from build123d import *

# Parameters (mm, degrees)
SKETCH2_R               = 10
BOSS_EXTRUDE1_DEPTH     = 70
CUT_EXTRUDE1_DEPTH      = 74.143694192
CUT_EXTRUDE1_DEPTH_BACK = 74.143694192


with BuildPart() as part:
    # Sketch1 → Revolve1 (revolve)
    with BuildSketch(Plane.XY):
        with BuildLine():
            Line((0, 15), (0, -15))
            ThreePointArc((0, -15), (15, 0), (0, 15))
        make_face()
    revolve(axis=Axis((0, -733.142524484, 0), (0, 1, 0)))

    # Sketch2 → Boss-Extrude1 (add)
    with BuildSketch(Plane(origin=(0, 0, 0), x_dir=(1, 0, 0), z_dir=(0, 1, 0))):
        with Locations(Location((0, 0, 0), (0, 0, 90))):
            Circle(SKETCH2_R)
    extrude(amount=BOSS_EXTRUDE1_DEPTH)

    # Sketch3 → Cut-Extrude1 (cut, two sides: drawn at the far end of the back side and taken through both)
    with BuildSketch(Plane.XY.offset(-CUT_EXTRUDE1_DEPTH_BACK)):
        Polygon((10, 45), (5, 35), (10, 25), align=None)
        Polygon((-10, 45), (-10, 25), (-5, 35), align=None)
    extrude(amount=CUT_EXTRUDE1_DEPTH + CUT_EXTRUDE1_DEPTH_BACK, mode=Mode.SUBTRACT)


solid = part.part
CAD build for the part. Positions are in the model's coordinates, mm. A direction names the side the tool comes from. Round coordinates to 2 decimals unless told otherwise and drop trailing zeros. Write each loop counter-clockwise with the first axis right and the second up, starting at its lowest first coordinate (ties: lowest second). Pieces come first, ordered by that corner, then holes. Notation, with made-up numbers: M 13.25,-37.5 L 64.25,-37.5 A19 ccw 64.25,-1.5 Z; hole C 70.5,76 d3. An arc over 180 degrees is marked long. Put each result on its own line as item: value. Start each with the question number.
1) 3-axis set-ups, long thin cutter, end or side, ignore diameter. For faces 1 (the flat face through (7, 39, 0)), 2 (the cylindrical face through (-3, 40.18, -9.54)), 3 (the flat face through (-7, 39, 0)): which of +Z, -Z, +X, -X, +Y, -Y reach the whole face in a straight line?
2) Pull direction Y, two halves, no side cores. Call faces 4 (the flat face through (7, 31, 0)), 5 (the flat face through (0, 70, 0)): pulls with the +Y half, pulls with the -Y half, needs draft (parallel to the pull), parting line crosses it, or undercut.
3) Pin check, flat tips, straight feed: pin 1 Ø10 at (x, z) = (-3.5, -10.5) entering from +Y; pin 2 Ø8 at (x, y) = (9, 22) entering from +Z; pin 3 Ø8 at (y, z) = (3.5, -3.5) entering from +X; pin 4 Ø10 at (x, y) = (5.5, 10.5) entering from -Z. Stop position of each tip, or through.
4) Drill centre lines: probe 1 along Y at (x, z) = (-9, 2); probe 2 along X at (y, z) = (24, 4.75); probe 3 along X at (y, z) = (3, -0.25). Where is each one in solid material? Low to high. Write a range as [from, to].
5) Saw through at C-C, the plane y = 46. Write the cut outline in (x, z).
6) Saw through at A-A, the plane x = -8.75. Write the cut outline in (y, z).
7) Saw through at D-D, the plane z = 5.75. Write the cut outline in (x, y), and give its area (3 significant figures).
8) Saw through at B-B, the plane z = 0. Write the cut outline in (x, y).
Resolved:
1. face 1: +Z, -Z, +X
1. face 2: +Y
1. face 3: +Z, -Z, -X
2. face 4: undercut
2. face 5: pulls with the +Y half
3. pin 1: y = 70
3. pin 2: z = 8.66
3. pin 3: x = 14.97
3. pin 4: z = -13.34
4. probe 1: [-11.83, 27], [43, 70]
4. probe 2: [-8.8, 8.8]
4. probe 3: [-14.69, 14.69]
5. outline: C 0,0 d20
6. outline: M 11.18,-4.84 L 27.5,-4.84 L 27.5,4.84 L 11.18,4.84 A12.18 ccw long Z; M 42.5,-4.84 L 70,-4.84 L 70,4.84 L 42.5,4.84 Z
7. outline: M -8.18,11.18 A13.85 ccw long 8.18,11.18 L 8.18,28.64 L 5,35 L 8.18,41.36 L 8.18,70 L -8.18,70 L -8.18,41.36 L -5,35 L -8.18,28.64 Z
7. area: 1,500 mm²
8. outline: M -10,11.18 A15 ccw long 10,11.18 L 10,25 L 5,35 L 10,45 L 10,70 L -10,70 L -10,45 L -5,35 L -10,25 Z
